Could you check a few things on this model? Use its own coordinates, in mm. Face numbers are marked on the shaded views. Coordinates: 2 decimals unless noted, no trailing zeros. Loops run counter-clockwise (first coordinate to the right, second up) from the corner with the lowest first, then second, coordinate; pieces in that order, holes last. Notation, with made-up numbers: (34, 57) - (93, 57) arc R29 cw to (93, 80) - close; hole circle Ø5 at (51.25, 83). An arc over 180 degrees is marked (long way). Use CSV: the item, a comma, the result in double quotes.
from build123d import *

# Parameters (mm, degrees)
SKETCH_1_R               = 11
EXTRUDE_1_DEPTH          = 2
SKETCH_2_R               = 5
EXTRUDE_2_DEPTH          = 10
SKETCH_3_R               = 3
CUT_EXTRUDE_1_DEPTH      = 20.646882704
SKETCH_4_R               = 1.5
CUT_EXTRUDE_2_DEPTH      = 20.646882704
PATTERN_CIRCULAR_1_COUNT = 4
FILLET_1_R               = 0.25


with BuildPart() as part:
    # ｽｹｯﾁ1 → ﾎﾞｽ - 押し出し1 (new body)
    with BuildSketch(Plane(origin=(0, 0, 0), x_dir=(1, 0, 0), z_dir=(0, 1, 0))):
        with Locations(Location((0, 0, 0), (0, 0, 270))):
            Circle(SKETCH_1_R)
    extrude(amount=EXTRUDE_1_DEPTH)

    # ｽｹｯﾁ2 → ﾎﾞｽ - 押し出し2 (add)
    with BuildSketch(Plane(origin=(0, 2, 0), x_dir=(1, 0, 0), z_dir=(0, 1, 0))):
        with Locations(Location((0, 0, 0), (0, 0, 270))):
            Circle(SKETCH_2_R)
    extrude(amount=EXTRUDE_2_DEPTH)

    # ｽｹｯﾁ3 → ｶｯﾄ - 押し出し1 (cut, through all)
    with BuildSketch(Plane(origin=(0, 12, 0), x_dir=(1, 0, 0), z_dir=(0, 1, 0))):
        with Locations(Location((0, 0, 0), (0, 0, 270))):
            Circle(SKETCH_3_R)
    extrude(amount=-CUT_EXTRUDE_1_DEPTH, mode=Mode.SUBTRACT)

    # ｽｹｯﾁ4 → ｶｯﾄ - 押し出し2 (cut, through all)
    with BuildSketch(Plane.XZ):
        with Locations(Location((0, 8, 0), (0, 0, 270))):
            Circle(SKETCH_4_R)
    cut_extrude_2 = extrude(amount=-CUT_EXTRUDE_2_DEPTH, mode=Mode.SUBTRACT)

    # 円形ﾊﾟﾀｰﾝ1: ｶｯﾄ - 押し出し2 ×4 about axis
    pattern_circular_1_axis = Axis((0, 0, 0), (0, 1, 0))
    for i in range(1, PATTERN_CIRCULAR_1_COUNT):
        add(cut_extrude_2.rotate(pattern_circular_1_axis, i * 360 / PATTERN_CIRCULAR_1_COUNT), mode=Mode.SUBTRACT)

    # ﾌｨﾚｯﾄ1
    fillet_1_edges = [part.edges().sort_by_distance(p)[0] for p in [
        (0, 0, -11),
        (0, 2, -11),
        (0, 2, -5),
        (0, 12, -5),
    ]]
    fillet(fillet_1_edges, radius=FILLET_1_R)


solid = part.part
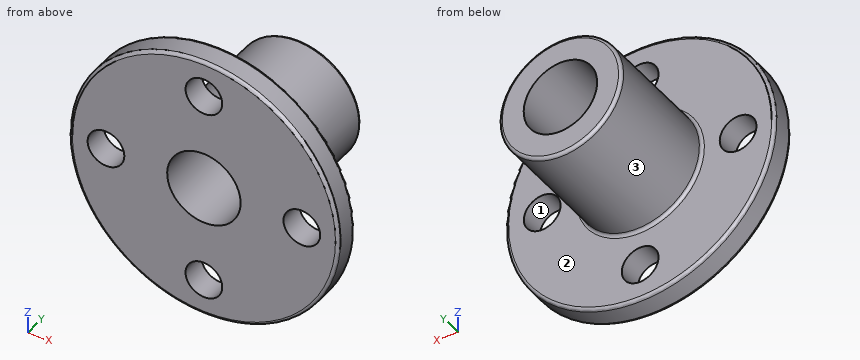
(1) Please list where these lines run through material, in increasing order: line 1 (Y direction, x = 4.5, z = -6.5); line 2 (X direction, y = 1.1, z = -8); line 3 (X direction, y = 9.5, z = -1).
Computed:
line 1,"y = 0 to 2"
line 2,"x = -7.55 to -1.5, 1.5 to 7.55"
line 3,"x = -4.9 to -2.83, 2.83 to 4.9"
(2) Suppose I cut it at B-B (z = 0). Write out the boundary of the cut face in (x, y), plus the area to 3 significant figures.
Computed:
outline,"(-11, 0.25) arc R0.25 ccw to (-10.75, 0) - (-9.5, 0) - (-9.5, 2) - (-10.75, 2) arc R0.25 ccw to (-11, 1.75) - close; (-6.5, 0) - (-3, 0) - (-3, 12) - (-4.75, 12) arc R0.25 ccw to (-5, 11.75) - (-5, 2.25) arc R0.25 cw to (-5.25, 2) - (-6.5, 2) - close; (3, 0) - (6.5, 0) - (6.5, 2) - (5.25, 2) arc R0.25 cw to (5, 2.25) - (5, 11.75) arc R0.25 ccw to (4.75, 12) - (3, 12) - close; (9.5, 0) - (10.75, 0) arc R0.25 ccw to (11, 0.25) - (11, 1.75) arc R0.25 ccw to (10.75, 2) - (9.5, 2) - close"
area,"59.9 mm²"
(3) Suppose I cut it at A-A (x = 0). Write out the boundary of the cut face in (y, z), plus the area to 3 significant figures.
Computed:
outline,"(0, -10.75) arc R0.25 ccw to (0.25, -11) - (1.75, -11) arc R0.25 ccw to (2, -10.75) - (2, -9.5) - (0, -9.5) - close; (0, -6.5) - (2, -6.5) - (2, -5.25) arc R0.25 cw to (2.25, -5) - (11.75, -5) arc R0.25 ccw to (12, -4.75) - (12, -3) - (0, -3) - close; (0, 3) - (12, 3) - (12, 4.75) arc R0.25 ccw to (11.75, 5) - (2.25, 5) arc R0.25 cw to (2, 5.25) - (2, 6.5) - (0, 6.5) - close; (0, 9.5) - (2, 9.5) - (2, 10.75) arc R0.25 ccw to (1.75, 11) - (0.25, 11) arc R0.25 ccw to (0, 10.75) - close"
area,"59.9 mm²"
(4) Suppose I cut it at C-C (y = 5.75). Write out the boundary of the cut face in (x, z).
Computed:
outline,"circle Ø10 at (0, 0); hole circle Ø6 at (0, 0)"
(5) Thinking about a two-plate mould opening in X: for the marked faces 1, 2 and 3, which applies, +X half, -X half, draft (parallel to the pull), parting line (faces both ways), or undercut?
Computed:
face 1,"undercut"
face 2,"draft"
face 3,"parting line"
(6) Will these pins go through, and if not, where does the flat tip stop? pin 1 (1.5 mm diameter, centred on x = -2.5, y = 10.5, fed in from +Z); pin 2 (4 mm diameter, centred on x = 2, y = 8.5, fed in from -Z); pin 3 (1.8 mm diameter, centred on x = 8, z = 0, fed in from +Y); pin 4 (2 mm diameter, centred on y = 8, z = 0.5, fed in from -X).
Computed:
pin 1,"stops at z = 4.68"
pin 2,"stops at z = -5"
pin 3,"passes through"
pin 4,"stops at x = -5"
